For this review, take the finished solid that the model builds, in its own axes (mm). A direction names the side the tool comes from. Give positions to 0.01 mm unless a question says otherwise; leave off trailing zeros. Write each loop counter-clockwise with the first axis right and the second up, starting at its lowest first coordinate (ties: lowest second). Pieces come first, ordered by that corner, then holes. Notation, with made-up numbers: M 41.5,-16.75 L 90.5,-16.75 A14 cw 90.5,0.25 Z; hole C 68,55 d4. An arc over 180 degrees is marked long. One line per item, written item: value. Start each with the question number.
Item 1: Tool access review of faces 1 (the face through (2, -5.05, 0)), 2 (the face through (0, -5.3, 0.2)), 3 (the face through (4.746, -10.855, 1.183)): name each direction out of +Z, -Z, +X, -X, +Y, -Y from which nothing blocks a thin tool from reaching the whole face with its end or side.
Item 2: Mouldability with a two-part tool opening along Y and no side actions: class faces 4 (the face through (2.46, 4.45, 4.48)), 5 (the face through (2.5, -1.5, 11.4)), 6 (the face through (5, -5.3, 0.2)) as released by +Y, released by -Y, zero draft, split by the parting line, or undercut.
Item 3: Consider section C-C, the plane z = -9. Write out the cut boundary in (x, y).
Item 4: Consider section D-D, the plane y = -9. Write out the cut boundary in (x, z).
Item 5: Consider section B-B, the plane y = -4. Write out the cut boundary in (x, z).
Item 6: Consider section A-A, the plane x = 4.05. Write out the cut boundary in (y, z).
Item 7: Clearance check with flat-ended pins moving along their axes: pin 1 Ø2 at (y, z) = (-2.5, 3) entering from -X; pin 2 Ø1.5 at (x, z) = (3.5, -1.5) entering from -Y; pin 3 Ø2.5 at (y, z) = (-9, 0) entering from +X; pin 4 Ø3 at (x, z) = (1.5, -5) entering from +Y. State where each tip first meets the part, or that it passes through.
Item 8: To check wall thickness, follow probe 1 along Z at (x, y) = (2.2, 0); probe 2 along Z at (x, y) = (0.85, -3.5); probe 3 along Y at (x, z) = (1.5, 1.25). State the ranges of each line that lie inside material, in increasing order.
```python
from build123d import *

# Parameters (mm, degrees)
F0_R     = 11.5
F0_R_2   = 1.05
F0_R_3   = 1
F1_DEPTH = 5


with BuildPart() as f1:
    # F0 (on Right) → F1 (new body)
    with BuildSketch(Plane.YZ):
        Circle(F0_R)
        with Locations((0, -9)):
            Circle(F0_R_2, mode=Mode.SUBTRACT)
        with Locations((-9, 0)):
            Circle(F0_R_3, mode=Mode.SUBTRACT)
        with BuildLine():
            ThreePointArc((-5.05, 3.05), (-4.464214, 4.464214), (-3.05, 5.05))
            Line((-3.05, 5.05), (3.05, 5.05))
            ThreePointArc((3.05, 5.05), (4.464214, 4.464214), (5.05, 3.05))
            Line((5.05, 3.05), (5.05, -3.05))
            ThreePointArc((5.05, -3.05), (4.464214, -4.464214), (3.05, -5.05))
            Line((3.05, -5.05), (-3.05, -5.05))
            ThreePointArc((-3.05, -5.05), (-4.464214, -4.464214), (-5.05, -3.05))
            Line((-5.05, -3.05), (-5.05, 3.05))
        make_face(mode=Mode.SUBTRACT)
        with Locations((9, 0)):
            Circle(F0_R_3, mode=Mode.SUBTRACT)
        with Locations((0, 9)):
            Circle(F0_R_2, mode=Mode.SUBTRACT)
    extrude(amount=F1_DEPTH)

    # F3 (on offset) → F5 (revolve, cut)
    with BuildSketch(Plane.XZ.offset(9)):
        Polygon((2.3, 0), (5, 0), (5, 2.2), (4.5, 2.2), align=None)
    revolve(axis=Axis((2.750115, -9, 0), (1, 0, 0)), mode=Mode.SUBTRACT)

    # F7 (on offset) → F8 (revolve, cut)
    with BuildSketch(Plane.XZ.offset(-9)):
        Polygon((4.5, 2.2), (2.3, 0), (5, 0), (5, 2.2), align=None)
    revolve(axis=Axis((3.65, 9, 0), (1, 0, 0)), mode=Mode.SUBTRACT)


solid = f1.part
```
Model answer:
1. face 1: +X, -X
1. face 2: +Z, -Z, -X, +Y, -Y
1. face 3: +X
2. face 4: undercut
2. face 5: split by the parting line
2. face 6: zero draft
3. outline: M 0,-7.16 L 5,-7.16 L 5,-1.05 L 0,-1.05 Z; M 0,1.05 L 5,1.05 L 5,7.16 L 0,7.16 Z
4. outline: M 0,-7.16 L 5,-7.16 L 5,-2.2 L 4.5,-2.2 L 3.3,-1 L 0,-1 Z; M 0,1 L 3.3,1 L 4.5,2.2 L 5,2.2 L 5,7.16 L 0,7.16 Z
5. outline: M 0,-10.78 L 5,-10.78 L 5,-4.81 L 0,-4.81 Z; M 0,4.81 L 5,4.81 L 5,10.78 L 0,10.78 Z
6. outline: C 0,0 d23; hole C -9,0 d3.5; hole M -5.05,-3.05 A2 ccw -3.05,-5.05 L 3.05,-5.05 A2 ccw 5.05,-3.05 L 5.05,3.05 A2 ccw 3.05,5.05 L -3.05,5.05 A2 ccw -5.05,3.05 Z; hole C 0,-9 d2.1; hole C 0,9 d2.1; hole C 9,0 d3.5
7. pin 1: passes through
7. pin 2: stops at y = -11.48
7. pin 3: stops at x = 3.55
7. pin 4: stops at y = 10.95
8. probe 1: z = -11.5 to -10.05, -7.95 to -5.05, 5.05 to 7.95, 10.05 to 11.5
8. probe 2: z = -10.95 to -5, 5 to 10.95
8. probe 3: y = -11.43 to -5.05, 5.05 to 11.43
